The drawing under review shows one solid part. Ordinate dimensions are in mm from its lowest x, y, z. A direction names the side the tool comes from. Coordinates: 2 decimals unless noted, no trailing zeros. Order: outer loops, then holes, each group sorted by start corner. A loop starts at its lowest first (then second) coordinate and runs counter-clockwise, first axis right, second up.
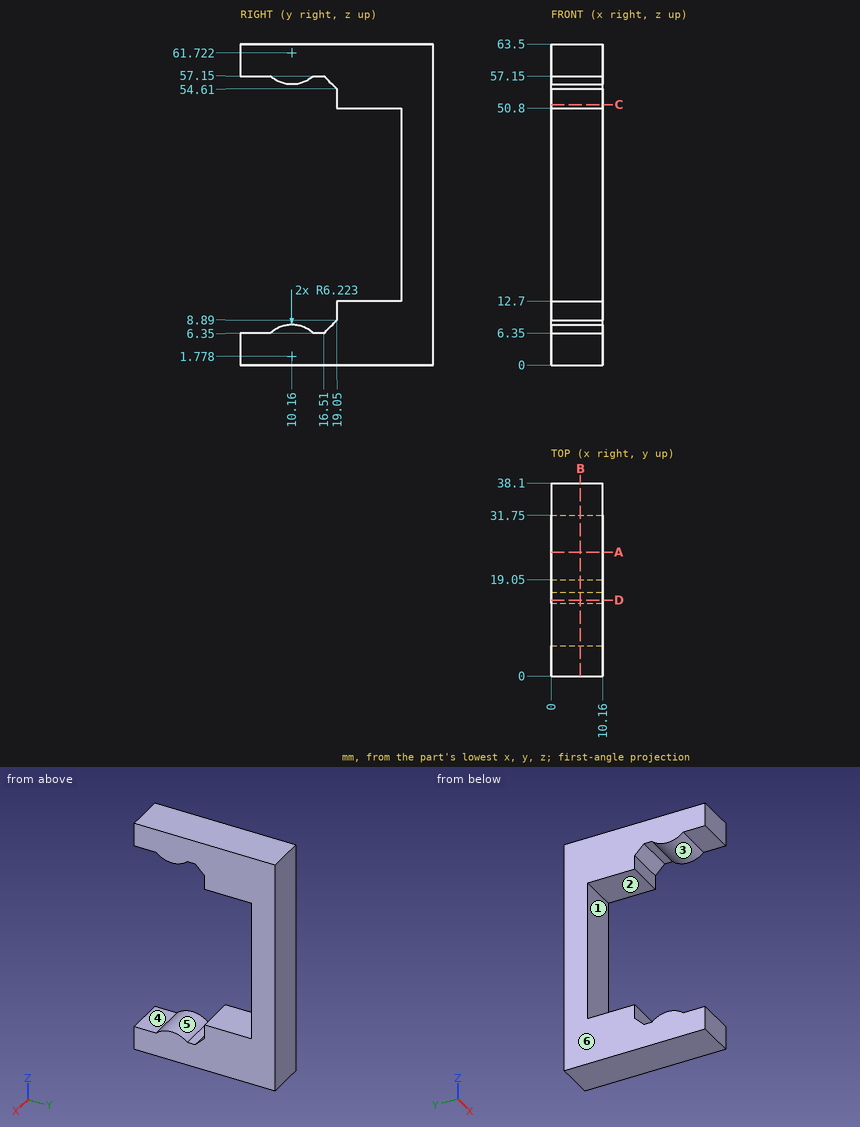
1. Take a section at C-C, the plane z = 51.5. Give the boundary of the cut face in (x, y).
Answer below:
outline: (0, 19.05) - (10.16, 19.05) - (10.16, 38.1) - (0, 38.1) - close
2. Take a section at D-D, the plane y = 15. Give the boundary of the cut face in (x, z), plus the area to 3 significant figures.
Answer below:
outline: (0, 0) - (10.16, 0) - (10.16, 6.35) - (0, 6.35) - close; (0, 57.15) - (10.16, 57.15) - (10.16, 63.5) - (0, 63.5) - close
area: 129 mm2
3. Take a section at B-B, the plane x = 5.75. Give the boundary of the cut face in (y, z), plus the area to 3 significant figures.
Answer below:
outline: (0, 0) - (38.1, 0) - (38.1, 63.5) - (0, 63.5) - (0, 57.15) - (5.94, 57.15) arc R6.22 ccw to (14.38, 57.15) - (16.51, 57.15) - (19.05, 54.61) - (19.05, 50.8) - (31.75, 50.8) - (31.75, 12.7) - (19.05, 12.7) - (19.05, 8.89) - (16.51, 6.35) - (14.38, 6.35) arc R6.22 ccw to (5.94, 6.35) - (0, 6.35) - close
area: 993 mm2
4. Machinability: for the marked faces 4, 5 and 6, which of the approach directions +Z, -Z, +X, -X, +Y, -Y give a long, thin tool a straight path to every point of the face, cutting with its end or side? Answer none if there is none.
Answer below:
face 4: +X, -X, -Y
face 5: +X, -X
face 6: +Z, -Z, -X, +Y, -Y
5. To check wall thickness, follow L1, parallel to Z at x = 3.25, y = 20; L2, parallel to Z at x = 2.25, y = 2.5; L3, parallel to Y at x = 7.75, z = 45. State the ranges of each line that lie inside material, in increasing order.
Answer below:
L1: z = 0 to 12.7, 50.8 to 63.5
L2: z = 0 to 6.35, 57.15 to 63.5
L3: y = 31.75 to 38.1
6. Take a section at A-A, the plane y = 24.5. Give the boundary of the cut face in (x, z).
Answer below:
outline: (0, 0) - (10.16, 0) - (10.16, 12.7) - (0, 12.7) - close; (0, 50.8) - (10.16, 50.8) - (10.16, 63.5) - (0, 63.5) - close
7. Clearance check with flat-ended pins moving along their axes: pin 1 Ø4 at (x, z) = (4, 53) entering from -Y; pin 2 Ø3 at (x, z) = (5, 37.5) entering from -Y. State where each tip first meets the part, or that it passes through.
Answer below:
pin 1: stops at y = 18.66
pin 2: stops at y = 31.75
8. The part is to be moulded in two halves that separate along Y. For the marked faces 1, 2 and 3, say which applies: +Y half, -Y half, draft (parallel to the pull), parting line (faces both ways), or undercut.
Answer below:
face 1: -Y half
face 2: draft
face 3: undercut
